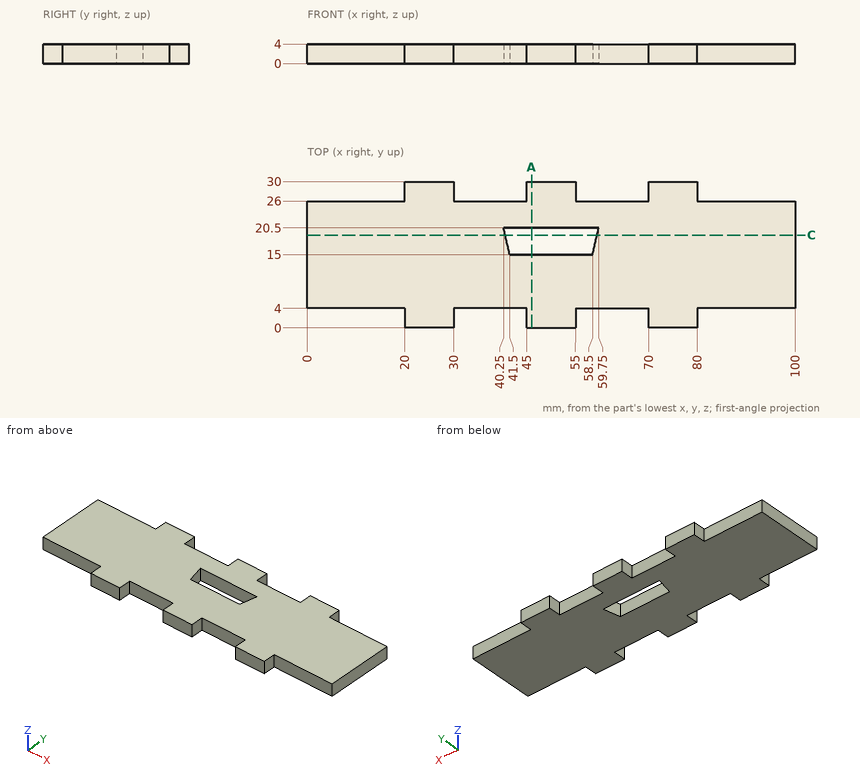
Part print with two shaded views. Sizes in mm from the minimum x, y, z corner. Give positions to 0.01 mm unless a question says otherwise; leave off trailing zeros. Order: outer loops, then holes, each group sorted by start corner. A loop starts at its lowest first (then second) coordinate and runs counter-clockwise, first axis right, second up.
(1) Drill centre lines: L1, parallel to X at y = 26.5, z = 0.8; L2, parallel to Y at x = 52, z = 2.25; L3, parallel to Y at x = 91, z = 0.55. Where is each one in solid material? Low to high.
(2) Saw through at A-A, the plane x = 46. Give the cut face in (y, z), then the cut area to 3 significant figures.
(3) Saw through at C-C, the plane y = 19. Give the cut face in (x, z).
(4) Flat gauge pins, fed straight in: pin 1 (2 mm diameter, centred on x = 35.5, z = 2.5, fed in from -Y); pin 2 (2 mm diameter, centred on y = 28.5, z = 2.5, fed in from +X); pin 3 (1.2 mm diameter, centred on y = 2.5, z = 2.5, fed in from -X). Where does each tip first touch, or does it go through?
Results found:
1. L1: x = 20 to 30, 45 to 55, 70 to 80
1. L2: y = 0 to 15, 20.5 to 30
1. L3: y = 4 to 26
2. outline: (0, 0) - (15, 0) - (15, 4) - (0, 4) - close; (20.5, 0) - (30, 0) - (30, 4) - (20.5, 4) - close
2. area: 98.0 mm2
3. outline: (0, 0) - (40.59, 0) - (40.59, 4) - (0, 4) - close; (59.41, 0) - (100, 0) - (100, 4) - (59.41, 4) - close
4. pin 1: stops at y = 4
4. pin 2: stops at x = 80
4. pin 3: stops at x = 20
